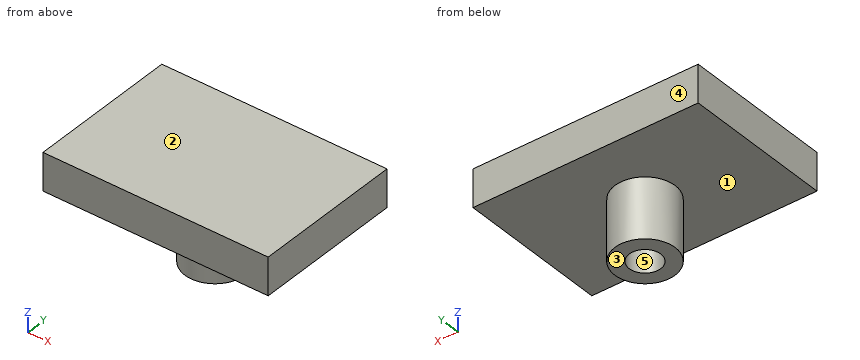
```python
from build123d import *

# Parameters (mm, degrees)
CROQUIS1_W              = 30
CROQUIS1_H              = 20
SALIENTE_EXTRUIR1_DEPTH = 5
CROQUIS2_R              = 4
SALIENTE_EXTRUIR3_DEPTH = 8
CROQUIS3_R              = 2.1
CORTAR_EXTRUIR1_DEPTH   = 6.5


with BuildPart() as part:
    # Croquis1 → Saliente-Extruir1 (new body)
    with BuildSketch(Plane.XY):
        Rectangle(CROQUIS1_W, CROQUIS1_H)
    extrude(amount=SALIENTE_EXTRUIR1_DEPTH)

    # Croquis2 → Saliente-Extruir3 (add)
    with BuildSketch(Plane(origin=(0, 0, 0), x_dir=(-1, 0, 0), z_dir=(0, 0, -1))):
        Circle(CROQUIS2_R)
    extrude(amount=SALIENTE_EXTRUIR3_DEPTH)

    # Croquis3 → Cortar-Extruir1 (cut)
    with BuildSketch(Plane(origin=(0, 0, -8), x_dir=(-1, 0, 0), z_dir=(0, 0, -1))):
        Circle(CROQUIS3_R)
    extrude(amount=-CORTAR_EXTRUIR1_DEPTH, mode=Mode.SUBTRACT)


solid = part.part
```
Geometry check sheet. Reference: the model listing, model coordinates, mm. Face numbers are marked on the shaded views. A direction names the side the tool comes from. Round coordinates to 2 decimals unless told otherwise and drop trailing zeros. Write each loop counter-clockwise with the first axis right and the second up, starting at its lowest first coordinate (ties: lowest second). Pieces come first, ordered by that corner, then holes. Notation, with made-up numbers: (43.5, 3.25) -> (59.5, 3.25) arc R18 cw to (59.5, 14.25) -> close; hole circle Ø3 at (27.5, 14). An arc over 180 degrees is marked (long way). Put each result on its own line as item: value.
1) Access from +Z, -Z, +X, -X, +Y, -Y to the whole of each face (thin tool, end or side, straight path). Record for the marked faces 1 and 2.
Recorded:
face 1: -Z
face 2: +Z, +X, -X, +Y, -Y
2) Cross-section at A-A, the plane y = 0. Enter the section's corners in (x, z), plus the area to 3 significant figures.
Recorded:
outline: (-15, 0) -> (-4, 0) -> (-4, -8) -> (-2.1, -8) -> (-2.1, -1.5) -> (2.1, -1.5) -> (2.1, -8) -> (4, -8) -> (4, 0) -> (15, 0) -> (15, 5) -> (-15, 5) -> close
area: 187 mm2
3) Cross-section at D-D, the plane x = 10.25. Enter the section's corners in (y, z).
Recorded:
outline: (-10, 0) -> (10, 0) -> (10, 5) -> (-10, 5) -> close
4) Release check for a two-part mould opening along Y. For the marked faces 3, 4 and 5 record: pulls with the +Y half, pulls with the -Y half, needs draft (parallel to the pull), parting line crosses it, or undercut.
Recorded:
face 3: needs draft
face 4: pulls with the +Y half
face 5: undercut
5) Cross-section at C-C, the plane z = -5.25. Enter the section's corners in (x, y), plus the area to 3 significant figures.
Recorded:
outline: circle Ø8 at (0, 0); hole circle Ø4.2 at (0, 0)
area: 36.4 mm2
6) Depth check by flat-ended pin: P1, Ø2, axis at x = 0.5, z = -4.5, coming from the +Y side; P2, Ø1.5, axis at x = -4, z = -2.5, coming from the -Y side; P3, Ø4, axis at x = 3.5, y = 5.5, coming from the -Z side. Enter the tip coordinate at first touch or a pass-through.
Recorded:
P1: stops at y = 4
P2: stops at y = -2.33
P3: stops at z = 0
7) Cross-section at B-B, the plane x = 0. Enter the section's corners in (y, z).
Recorded:
outline: (-10, 0) -> (-4, 0) -> (-4, -8) -> (-2.1, -8) -> (-2.1, -1.5) -> (2.1, -1.5) -> (2.1, -8) -> (4, -8) -> (4, 0) -> (10, 0) -> (10, 5) -> (-10, 5) -> close
8) Thickness scan on probe 1 along Y at (x, z) = (0, -6.5); probe 2 along Z at (x, y) = (5.75, 0.75); probe 3 along X at (y, z) = (1.5, -5.5). Record the ranges inside material, lowest first. Write a range as from..to.
Recorded:
probe 1: y = -4..-2.1, 2.1..4
probe 2: z = 0..5
probe 3: x = -3.71..-1.47, 1.47..3.71
